from build123d import *

# Parameters (mm, degrees)
SKETCH3_W                                       = 90.422573022
SKETCH3_H                                       = 121.412
BOSS_EXTRUDE4_DEPTH                             = 2.54
BOSS_EXTRUDE5_DEPTH                             = 30.48
CUT_EXTRUDE2_DEPTH                              = 122.412
BOSS_EXTRUDE6_DEPTH                             = 33.02
SKETCH9_W                                       = 10.16
SKETCH9_H                                       = 23.622
CUT_EXTRUDE3_DEPTH                              = 27.94
BOSS_EXTRUDE7_DEPTH                             = 2.54
SKETCH12_W                                      = 23.622
SKETCH12_H                                      = 3.81
CUT_EXTRUDE4_DEPTH                              = 10.16
SKETCH13_W                                      = 12.7
SKETCH13_H                                      = 3.81
CUT_EXTRUDE5_DEPTH                              = 13.461069207
BOSS_EXTRUDE9_REACH                             = 62.706
BOSS_EXTRUDE9_DIRECTION_2_REACH                 = 62.706
CBORE_FOR_6_PAN_HEAD_MACHINE_SCREW1_D           = 3.6576
CBORE_FOR_6_PAN_HEAD_MACHINE_SCREW1_CBORE_D     = 7.54126
CBORE_FOR_6_PAN_HEAD_MACHINE_SCREW1_CBORE_DEPTH = 2.4638
F_6_CLEARANCE_HOLE1_D                           = 3.6576
SKETCH21_W                                      = 43.815
SKETCH21_H                                      = 22.86
CUT_EXTRUDE6_DEPTH                              = 33.781069207
CHAMFER1_SIZE                                   = 2.54
CHAMFER2_SIZE                                   = 3.81
SKETCH23_W                                      = 10.16
SKETCH23_H                                      = 23.622
CUT_EXTRUDE8_DEPTH                              = 0.762
CHAMFER3_SIZE                                   = 0.762


with BuildPart() as part:
    # Sketch3 → Boss-Extrude4 (new body)
    with BuildSketch(Plane(origin=(0, 0, 0), x_dir=(1, 0, 0), z_dir=(0, 1, 0))):
        Rectangle(SKETCH3_W, SKETCH3_H)
    extrude(amount=BOSS_EXTRUDE4_DEPTH)

    # Sketch6 → Boss-Extrude5 (add)
    with BuildSketch(Plane(origin=(0, 2.54, 0), x_dir=(1, 0, 0), z_dir=(0, 1, 0))):
        Polygon((45.211286511, -60.706), (45.211286511, 60.706), (-45.211286511, 60.706), (-45.211286511, 58.166), (42.671286511, 58.166), (42.671286511, -58.166), (-45.211286511, -58.166), (-45.211286511, -60.706), align=None)
    extrude(amount=BOSS_EXTRUDE5_DEPTH)

    # Sketch7 → Cut-Extrude2 (cut, through all)
    with BuildSketch(Plane.XY.offset(60.706)):
        Polygon((-42.671286511, 2.54), (-27.431286511, 17.78), (27.431286511, 17.78), (42.671286511, 33.02), (-45.211286511, 33.02), (-45.211286511, 2.54), align=None)
    extrude(amount=-CUT_EXTRUDE2_DEPTH, mode=Mode.SUBTRACT)

    # Sketch8 → Boss-Extrude6 (add)
    with BuildSketch(Plane(origin=(0, 0, 0), x_dir=(1, 0, 0), z_dir=(0, 1, 0))):
        Polygon((45.211286511, 14.351), (70.694027546, 14.351), (74.922106204, 10.122921342), (75.452355719, 6.35), (70.677155719, 6.35), (70.677155719, -6.35), (75.452355719, -6.35), (74.922106204, -10.122921342), (70.694027546, -14.351), (45.211286511, -14.351), align=None)
    extrude(amount=BOSS_EXTRUDE6_DEPTH)

    # Sketch9 → Cut-Extrude3 (cut)
    with BuildSketch(Plane(origin=(0, 33.02, 0), x_dir=(1, 0, 0), z_dir=(0, 1, 0))):
        with Locations((47.751286511, 0)):
            Rectangle(SKETCH9_W, SKETCH9_H)
    extrude(amount=-CUT_EXTRUDE3_DEPTH, mode=Mode.SUBTRACT)

    # Sketch11 → Boss-Extrude7 (add)
    with BuildSketch(Plane(origin=(0, 2.54, 0), x_dir=(1, 0, 0), z_dir=(0, 1, 0))):
        Polygon((35.051286511, 58.166), (27.431286511, 58.166), (29.971286511, 55.626), (32.511286511, 55.626), align=None)
        Polygon((-29.971286511, 55.626), (-32.511286511, 55.626), (-35.051286511, 58.166), (-27.431286511, 58.166), align=None)
        Polygon((29.971286511, -55.626), (32.511286511, -55.626), (35.051286511, -58.166), (27.431286511, -58.166), align=None)
        Polygon((-27.431286511, -58.166), (-29.971286511, -55.626), (-32.511286511, -55.626), (-35.051286511, -58.166), align=None)
    extrude(amount=BOSS_EXTRUDE7_DEPTH)

    # Sketch12 → Cut-Extrude4 (cut)
    with BuildSketch(Plane.ZY.offset(-52.831286511)):
        with Locations((0, 27.305)):
            Rectangle(SKETCH12_W, SKETCH12_H)
    extrude(amount=-CUT_EXTRUDE4_DEPTH, mode=Mode.SUBTRACT)

    # Sketch13 → Cut-Extrude5 (cut, through all)
    with BuildSketch(Plane.ZY.offset(-62.991286511)):
        with Locations((0, 27.305)):
            Rectangle(SKETCH13_W, SKETCH13_H)
    extrude(amount=-CUT_EXTRUDE5_DEPTH, mode=Mode.SUBTRACT)

    # Boss-Extrude9: up to this face of the body (flat: up to its plane)
    boss_extrude9_end = Plane(part.part.faces().sort_by_distance((48.970486511, 20.0406, -11.811))[0])
    # Sketch15 → Boss-Extrude9 (add, up to the picked face)
    with BuildSketch(Plane.XY, mode=Mode.PRIVATE) as boss_extrude9_sk1:
        Polygon((-62.991286511, 10.16), (-52.831286511, 10.16), (-45.211286511, 5.08), (-35.051286511, 5.08), (-35.051286511, 2.54), (-45.211286511, 2.54), (-45.211286511, 0), (-52.831286511, 0), (-52.831286511, 6.35), (-62.991286511, 6.35), align=None)
    boss_extrude9_tool1 = split(extrude(boss_extrude9_sk1.sketch, amount=-BOSS_EXTRUDE9_REACH, mode=Mode.PRIVATE), bisect_by=boss_extrude9_end, keep=Keep.BOTH, mode=Mode.PRIVATE)
    add(boss_extrude9_tool1.solids().sort_by_distance((-50.157602, 5.280526, 0))[0])

    # Boss-Extrude9 direction 2: up to this face of the body (flat: up to its plane)
    boss_extrude9_direction_2_end = Plane(part.part.faces().sort_by_distance((48.970486511, 20.0406, 11.811))[0])
    # Sketch15 → Boss-Extrude9 direction 2 (add, up to the picked face)
    with BuildSketch(Plane.XY, mode=Mode.PRIVATE) as boss_extrude9_direction_2_sk1:
        Polygon((-62.991286511, 10.16), (-52.831286511, 10.16), (-45.211286511, 5.08), (-35.051286511, 5.08), (-35.051286511, 2.54), (-45.211286511, 2.54), (-45.211286511, 0), (-52.831286511, 0), (-52.831286511, 6.35), (-62.991286511, 6.35), align=None)
    boss_extrude9_direction_2_tool1 = split(extrude(boss_extrude9_direction_2_sk1.sketch, amount=BOSS_EXTRUDE9_DIRECTION_2_REACH, mode=Mode.PRIVATE), bisect_by=boss_extrude9_direction_2_end, keep=Keep.BOTH, mode=Mode.PRIVATE)
    add(boss_extrude9_direction_2_tool1.solids().sort_by_distance((-50.157602, 5.280526, 0))[0])

    # CBORE for #6 Pan Head Machine Screw1 (through all)
    with Locations(Plane(origin=(0, 0, 0), x_dir=(-1, 0, 0), z_dir=(0, -1, 0))):
        with Locations((-47.751286511, 6.731), (-47.751286511, -6.731), (40.131286511, 6.731), (40.131286511, -6.731)):
            CounterBoreHole(CBORE_FOR_6_PAN_HEAD_MACHINE_SCREW1_D / 2, CBORE_FOR_6_PAN_HEAD_MACHINE_SCREW1_CBORE_D / 2, CBORE_FOR_6_PAN_HEAD_MACHINE_SCREW1_CBORE_DEPTH)

    # #6 Clearance Hole1 (through all)
    with Locations(Plane(origin=(0, 33.02, 0), x_dir=(1, 0, 0), z_dir=(0, 1, 0))):
        with Locations((-57.911286511, 0), (57.911286511, 0)):
            Hole(F_6_CLEARANCE_HOLE1_D / 2)

    # Sketch21 → Cut-Extrude6 (cut, through all)
    with BuildSketch(Plane.ZY.offset(-42.671286511)):
        with Locations((-36.2585, 17.78)):
            Rectangle(SKETCH21_W, SKETCH21_H)
        with Locations((36.2585, 17.78)):
            Rectangle(SKETCH21_W, SKETCH21_H)
    extrude(amount=-CUT_EXTRUDE6_DEPTH, mode=Mode.SUBTRACT)

    # Chamfer1
    chamfer1_edges = [part.edges().sort_by_distance(p)[0] for p in [
        (-52.831286511, 0, 0),
        (-35.051286511, 3.81, -11.811),
        (-62.991286511, 8.255, -11.811),
        (-62.991286511, 8.255, 11.811),
        (-35.051286511, 3.81, 11.811),
    ]]
    chamfer(chamfer1_edges, length=CHAMFER1_SIZE)

    # Chamfer2
    chamfer2_edges = [part.edges().sort_by_distance(p)[0] for p in [
        (45.211286511, 3.175, -14.351),
        (45.211286511, 3.175, 14.351),
        (45.211286511, 31.115, -14.351),
        (45.211286511, 31.115, 14.351),
    ]]
    chamfer(chamfer2_edges, length=CHAMFER2_SIZE)

    # Sketch23 → Cut-Extrude8 (cut)
    with BuildSketch(Plane.XZ.offset(-6.35)):
        with Locations((-57.911286511, 0)):
            Rectangle(SKETCH23_W, SKETCH23_H)
    extrude(amount=-CUT_EXTRUDE8_DEPTH, mode=Mode.SUBTRACT)

    # Chamfer3
    chamfer3_edges = [part.edges().sort_by_distance(p)[0] for p in [
        (-62.991286511, 10.16, 0),
        (-62.991286511, 7.112, 0),
    ]]
    chamfer(chamfer3_edges, length=CHAMFER3_SIZE)


solid = part.part
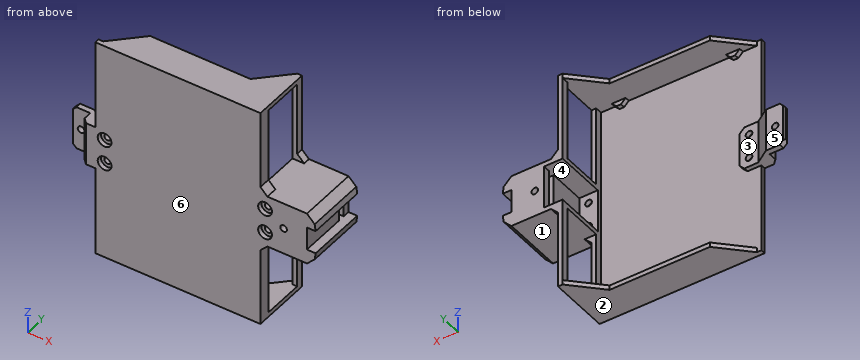
Geometry check sheet. Reference: the model listing, model coordinates, mm. Face numbers are marked on the shaded views. A direction names the side the tool comes from. Give positions to 0.01 mm unless a question says otherwise; leave off trailing zeros. Loops run counter-clockwise (first coordinate to the right, second up) from the corner with the lowest first, then second, coordinate; pieces in that order, holes last. Notation, with made-up numbers: M 42,-38.75 L 50,-38.75 A20 ccw 50,-6.75 Z; hole C 83,48 d9. An arc over 180 degrees is marked long. Write each question's results on one line, items separated by ' | '.
1) Section check D-D, the plane x = -12. Record the boundary of the cut face in (y, z), plus the area to 3 significant figures.
Answers follow:
outline: M 0,-60.71 L 17.78,-60.71 L 17.78,-58.17 L 2.54,-58.17 L 2.54,58.17 L 17.78,58.17 L 17.78,60.71 L 0,60.71 Z | area: 386 mm2
2) Section check C-C, the plane z = 0. Count the separate pieces of the cut face and the enclosed holes in it, plus the area to 3 significant figures.
Answers follow:
separate pieces: 5 | enclosed holes: 0 | area: 789 mm2
3) Release check for a two-part mould opening along Y. For the marked faces 1, 2 and 3 record: +Y half, -Y half, draft (parallel to the pull), parting line (faces both ways), or undercut.
Answers follow:
face 1: undercut | face 2: draft | face 3: +Y half
4) Gauge pin test, flat ends, axial feed: pin 1 (3 mm diameter, centred on y = 29, z = -19, fed in from -X); pin 2 (0.8 mm diameter, centred on y = 4, z = 0.5, fed in from +X); pin 3 (8.5 mm diameter, centred on x = 60, y = 22.5, fed in from -Z). Record the tip position at first contact, or that the pin passes through.
Answers follow:
pin 1: x = 42.67 | pin 2: x = 70.68 | pin 3: z = -14.35
5) Section check A-A, the plane y = 13. Record the boundary of the cut face in (x, z).
Answers follow:
outline: M -32.21,-60.71 L 45.21,-60.71 L 45.21,-58.17 L -32.21,-58.17 Z; M -32.21,58.17 L 45.21,58.17 L 45.21,60.71 L -32.21,60.71 Z; M 42.67,-14.35 L 70.69,-14.35 L 74.92,-10.12 L 75.45,-6.35 L 70.68,-6.35 L 70.68,6.35 L 75.45,6.35 L 74.92,10.12 L 70.69,14.35 L 42.67,14.35 L 42.67,11.81 L 52.83,11.81 L 52.83,-11.81 L 42.67,-11.81 Z; hole C 57.91,0 d3.66
6) Tool access check on the marked faces 4, 5 and 6. Record the directions out of +Z, -Z, +X, -X, +Y, -Y that give a thin tool (end or side, any length) a straight path to the whole face; none if there is none.
Answers follow:
face 4: none | face 5: +Z, -Z, -X, +Y | face 6: +Z, -Z, +X, -X, -Y
7) Thickness scan on line 1 (Z direction, x = 40.5, y = 6.5); line 2 (Y direction, x = 40, z = 10); line 3 (X direction, y = 31, z = 26). Record the ranges inside material, lowest first.
Answers follow:
line 1: -60.71 to -58.17, 58.17 to 60.71 | line 2: 0 to 2.54 | line 3: 42.67 to 45.21
8) Section check B-B, the plane z = 34.5. Record the boundary of the cut face in (x, y), plus the area to 3 significant figures.
Answers follow:
outline: M -45.21,0 L 45.21,0 L 45.21,6.35 L 42.67,6.35 L 42.67,2.54 L -45.21,2.54 Z; M 42.67,29.21 L 45.21,29.21 L 45.21,33.02 L 42.67,33.02 Z | area: 249 mm2
